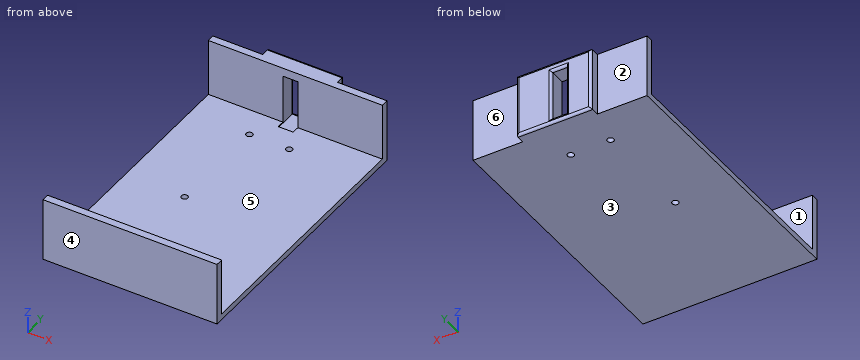
Autodesk Inventor part; units mm, degrees
ref_plane "YZ Plane" through (0, 0, 0) normal (1, 0, 0) x (0, 1, 0)
ref_plane "XZ Plane" through (0, 0, 0) normal (0, 1, 0) x (-1, 0, 0)
ref_plane "XY Plane" through (0, 0, 0) normal (0, 0, 1) x (1, 0, 0)
sketch "Sketch1" plane through (0, 0, 0) normal (0, 0, 1) x (1, 0, 0)
  line L0 (0, 0) -> (350, 0)
  line L1 (350, 0) -> (350, 520)
  line L2 (350, 520) -> (0, 520)
  line L3 (0, 520) -> (0, 0)
  dimension "d0" = 350
  dimension "d1" = 520
extrude "Extrusion1" add sketch "Sketch1" along normal blind 12
sketch "Sketch2" plane through (0, 0, 12) normal (0, 0, 1) x (1, 0, 0)
  line L0 (0, 120) -> (350, 120)
  line L1 (350, 120) -> (350, 370)
  line L2 (350, 0) -> (350, 520)
  line L3 (350, 370) -> (0, 370)
  line L4 (0, 520) -> (0, 0)
  line L5 (0, 370) -> (0, 520)
  line L6 (350, 520) -> (0, 520)
  line L7 (0, 520) -> (350, 520)
  line L8 (350, 520) -> (350, 370)
  circle A0 centre (120, 460) radius 6.5
  circle A1 centre (120, 250) radius 6.5
  dimension "d6" = 13
  dimension "d7" = 13
extrude "Extrusion2" cut sketch "Sketch2" against normal blind 12 contours A0 | A1
thread "Thread1"
thread "Thread2"
sketch "Sketch3" plane through (0, 0, 0) normal (0, 0, -1) x (-1, 0, 0)
  circle A0 centre (-200, 460) radius 6.5
  point P0 (0, 0)
  dimension "d14" = 13
extrude "Extrusion3" cut sketch "Sketch3" against normal blind 120
sketch "Sketch4" plane through (0, 520, 0) normal (0, 1, 0) x (1, 0, 0)
  line L0 (0, 0) -> (350, 0)
  line L1 (350, 0) -> (350, -12)
  line L2 (0, 0) -> (350, 0)
  line L3 (350, 0) -> (350, -12)
  line L4 (350, -12) -> (0, -12)
  line L5 (0, -12) -> (0, 0)
extrude "Extrusion4" add sketch "Sketch4" along normal blind 15
sketch "Sketch5" plane through (0, 0, 12) normal (0, 0, 1) x (1, 0, 0)
  line L0 (0, 0) -> (0, 535)
  line L1 (0, 535) -> (350, 535)
  line L2 (350, 535) -> (350, 520)
  line L3 (350, 520) -> (0, 520)
  line L4 (0, 520) -> (0, 535)
  dimension "d19" = 350
  dimension "d20" = 15
extrude "Extrusion5" add sketch "Sketch5" along normal blind 80
sketch "Sketch6" plane through (0, 0, 0) normal (0, -1, 0) x (1, 0, 0)
  line L0 (350, 0) -> (0, 0)
  line L1 (350, 12) -> (0, 12)
  line L2 (0, 0) -> (350, 0)
  line L3 (350, 0) -> (350, 12)
  line L4 (350, 12) -> (0, 12)
  line L5 (0, 12) -> (0, 0)
  dimension "d23" = 350
extrude "Extrusion6" add sketch "Sketch6" along normal blind 15
sketch "Sketch7" plane through (0, 0, 12) normal (0, 0, 1) x (1, 0, 0)
  line L0 (0, 0) -> (350, 0)
  line L1 (350, 0) -> (350, -15)
  line L2 (350, -15) -> (0, -15)
  line L3 (0, -15) -> (0, 0)
extrude "Extrusion7" add sketch "Sketch7" along normal blind 80
sketch "Sketch8" plane through (0, 0, 92) normal (0, 0, 1) x (1, 0, 0)
  line L0 (0, -15) -> (350, -15)
  line L1 (0, 0) -> (350, 0)
  line L2 (350, 0) -> (350, -15)
  line L3 (350, -15) -> (0, -15)
  line L4 (0, -15) -> (0, 0)
  line L5 (0, 535) -> (0, 520)
  line L6 (0, 520) -> (350, 520)
  line L7 (0, 535) -> (350, 535)
  line L8 (350, 535) -> (350, 520)
  line L9 (350, 520) -> (0, 520)
  line L10 (0, 520) -> (0, 535)
extrude "Extrusion8" add sketch "Sketch8" along normal blind 35
sketch "Sketch9" plane through (0, -15, 0) normal (0, -1, 0) x (1, 0, 0)
  point P0 (0, 0)
sketch "Sketch10" plane through (0, 535, 0) normal (0, 1, 0) x (1, 0, 0)
  line L0 (0, 0) -> (350, 0)
  line L1 (100, 0) -> (250, 0)
  line L2 (250, 0) -> (250, -127)
  line L3 (250, -127) -> (100, -127)
  line L4 (100, -127) -> (100, 0)
  dimension "d30" = 150
  dimension "d31" = 127
extrude "Extrusion9" add sketch "Sketch10" along normal blind 20
sketch "Sketch11" plane through (0, 555, 0) normal (0, 1, 0) x (1, 0, 0)
  point P0 (0, 0)
sketch "Sketch12" plane through (0, 555, 0) normal (0, 1, 0) x (1, 0, 0)
  point P0 (0, 0)
sketch "Sketch13" plane through (0, 555, 0) normal (0, 1, 0) x (1, 0, 0)
  line L0 (150, -110) -> (180, -110)
  line L1 (180, -110) -> (180, -10)
  line L2 (180, -10) -> (150, -10)
  line L3 (150, -10) -> (150, -110)
  point P0 (0, 0)
  dimension "d34" = 30
  dimension "d35" = 100
extrude "Extrusion10" cut sketch "Sketch13" against normal blind 50
fillet "Fillet1" radius 5 8 edges at (180, 555, 60) (150, 555, 60) (165, 555, 110) (165, 555, 10) (175, 555, 127) (250, 555, 63.5) (175, 555, 0) (100, 555, 63.5)
properties part number "back plate"
Geometry: final body of the model. Coordinates: model frame, mm. Face numbers are marked on the shaded views. A direction names the side the tool comes from. Coordinates: 2 decimals unless noted, no trailing zeros. Order: outer loops, then holes, each group sorted by start corner. A loop starts at its lowest first (then second) coordinate and runs counter-clockwise, first axis right, second up.
1) Section D-D (x = 200). Return loops of the section in (y, z), then the cut area to 3 significant figures.
Result sheet:
outline: (-15, 0) - (453.5, 0) - (453.5, 12) - (0, 12) - (0, 127) - (-15, 127) - close; (466.5, 0) - (550, 0) arc R5 ccw to (555, 5) - (555, 122) arc R5 ccw to (550, 127) - (520, 127) - (520, 12) - (466.5, 12) - close
area: 12,400 mm2
2) Ray query, probe 1 along Y at (x, z) = (120, 4); probe 2 along Y at (x, z) = (120, 7.75); probe 3 along Y at (x, z) = (230, 65). Return the intervals inside material, ascending.
Result sheet:
probe 1: y = -15 to 243.5, 256.5 to 453.5, 466.5 to 554.9
probe 2: y = -15 to 243.5, 256.5 to 453.5, 466.5 to 555
probe 3: y = -15 to 0, 520 to 555
3) Section B-B (x = 120). Return loops of the section in (y, z), then the cut area to 3 significant figures.
Result sheet:
outline: (-15, 0) - (243.5, 0) - (243.5, 12) - (0, 12) - (0, 127) - (-15, 127) - close; (256.5, 0) - (453.5, 0) - (453.5, 12) - (256.5, 12) - close; (466.5, 0) - (550, 0) arc R5 ccw to (555, 5) - (555, 122) arc R5 ccw to (550, 127) - (520, 127) - (520, 12) - (466.5, 12) - close
area: 12,300 mm2
4) First-contact query: P1, Ø0.6, axis at x = 159.5, z = 11.5, coming from the +Y side; P2, Ø1.5, axis at x = 51, z = 83.5, coming from the +Y side; P3, Ø7.5, axis at y = 544, z = 89, coming from the +X side. Flat tips, straight axial feed; report the tip coordinate or a pass-through.
Result sheet:
P1: stops at y = 505
P2: stops at y = 535
P3: stops at x = 250
5) Set-up query: the marked faces 4, 5 and 6. Return all of +Z, -Z, +X, -X, +Y, -Y with unobstructed straight access to the full face (end or side cutting, diameter ignored); none if empty.
Result sheet:
face 4: +Z, -Z, +X, -X, -Y
face 5: +Z, +X, -X
face 6: +Z, -Z, +X, +Y
6) Section C-C (z = 28.5). Return loops of the section in (x, y), then the cut area to 3 significant figures.
Result sheet:
outline: (0, -15) - (350, -15) - (350, 0) - (0, 0) - close; (0, 520) - (150, 520) - (150, 550) arc R5 ccw to (145, 555) - (105, 555) arc R5 ccw to (100, 550) - (100, 535) - (0, 535) - close; (180, 520) - (350, 520) - (350, 535) - (250, 535) - (250, 550) arc R5 ccw to (245, 555) - (185, 555) arc R5 ccw to (180, 550) - close
area: 12,400 mm2
7) Section A-A (y = 460). Return loops of the section in (x, z), then the cut area to 3 significant figures.
Result sheet:
outline: (0, 0) - (113.5, 0) - (113.5, 12) - (0, 12) - close; (126.5, 0) - (193.5, 0) - (193.5, 12) - (126.5, 12) - close; (206.5, 0) - (350, 0) - (350, 12) - (206.5, 12) - close
area: 3,890 mm2
8) Draft query along Y for the marked faces 1, 2 and 3. Return one class per face: released by +Y, released by -Y, zero draft, split by the parting line, or undercut.
Result sheet:
face 1: undercut
face 2: released by +Y
face 3: zero draft
